Study the drawing (mm; zero at the part's minimum x, y, z) and answer. A direction names the side the tool comes from. Coordinates: 2 decimals unless noted, no trailing zeros. Order: outer loops, then holes, each group sorted by start corner. A loop starts at its lowest first (then second) coordinate and runs counter-clockwise, first axis right, second up.
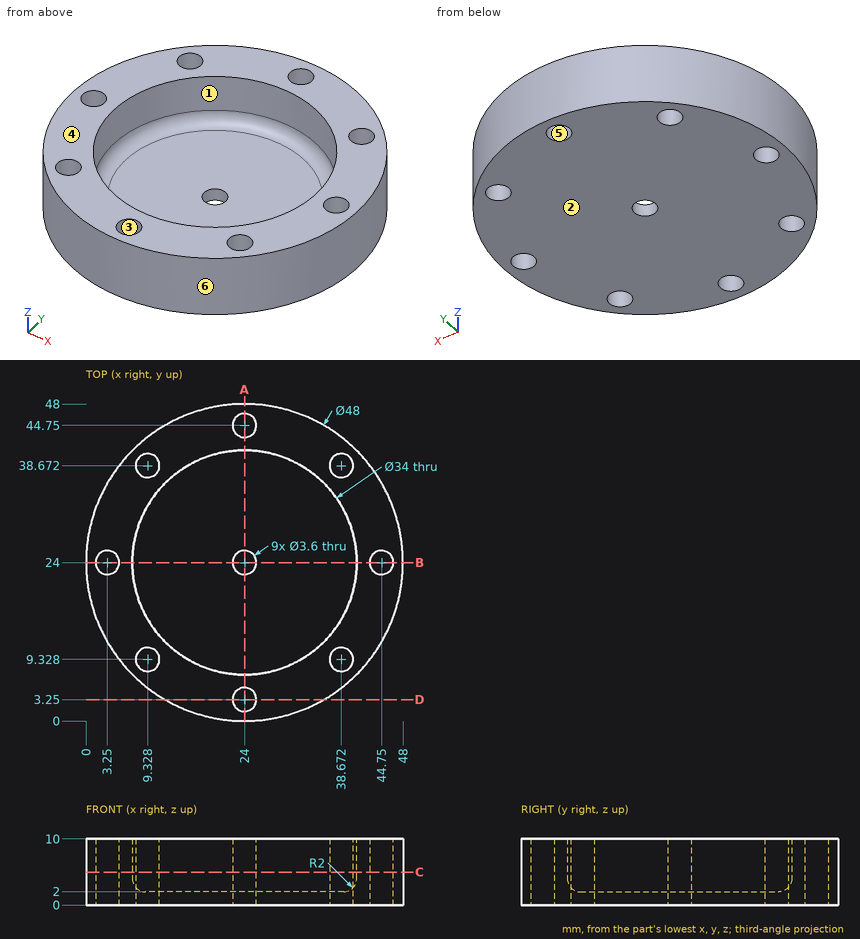
1) Determine the mould class of the marked faces 3, 4, 5 and 6 for opening direction Y: pulls with the +Y half, pulls with the -Y half, needs draft (parallel to the pull), parting line crosses it, or undercut.
A:
face 3: undercut
face 4: needs draft
face 5: undercut
face 6: parting line crosses it
2) Which of the six approach directions +Z, -Z, +X, -X, +Y, -Y give full straight-line access (tool end or side, diameter ignored) to the marked faces 1 and 2?
A:
face 1: +Z
face 2: -Z, +X, -X, +Y, -Y
3) Flat-ended cylindrical pins translate along their axes: pin 1 Ø3 at (x, y) = (44.75, 24) entering from -Z; pin 2 Ø4 at (x, z) = (9.5, 9) entering from +Y; pin 3 Ø3 at (x, z) = (36, 2) entering from +Y; pin 4 Ø1 at (x, y) = (17.5, 27.5) entering from +Z. Find the tip coordinate at first contact, or state that the pin passes through.
A:
pin 1: passes through
pin 2: stops at y = 44.49
pin 3: stops at y = 45.58
pin 4: stops at z = 2
4) A cutting plane is placed at A-A, the plane x = 24. Determine the outline of the cut face in (y, z).
A:
outline: (0, 0) - (1.45, 0) - (1.45, 10) - (0, 10) - close; (5.05, 0) - (22.2, 0) - (22.2, 2) - (9, 2) arc R2 cw to (7, 4) - (7, 10) - (5.05, 10) - close; (25.8, 0) - (42.95, 0) - (42.95, 10) - (41, 10) - (41, 4) arc R2 cw to (39, 2) - (25.8, 2) - close; (46.55, 0) - (48, 0) - (48, 10) - (46.55, 10) - close
5) A cutting plane is placed at D-D, the plane y = 3.25. Determine the outline of the cut face in (x, z), and give its area (3 significant figures).
A:
outline: (11.94, 0) - (22.2, 0) - (22.2, 10) - (11.94, 10) - close; (25.8, 0) - (36.06, 0) - (36.06, 10) - (25.8, 10) - close
area: 205 mm2
6) A cutting plane is placed at C-C, the plane z = 5. State how many separate pieces and enclosed holes the cut face has.
A:
separate pieces: 1
enclosed holes: 9
7) Straight lines are drawn through the part: line 1 (Y direction, x = 24, z = 1.2); line 2 (Y direction, x = 9.5, z = 3.25) (1 decimal); line 3 (Z direction, x = 19, y = 26.5). For each, find the intervals that lie inside material, in ascending order.
A:
line 1: y = 0 to 1.45, 5.05 to 22.2, 25.8 to 42.95, 46.55 to 48
line 2: y = 4.9 to 7.5, 11.1 to 15.4, 32.6 to 36.9, 40.5 to 43.1
line 3: z = 0 to 2
